Answer from the drawing. Dimensions are ordinates in mm from the lowest x, y and z of the part. Coordinates: 2 decimals unless noted, no trailing zeros. Order: outer loops, then holes, each group sorted by start corner. A loop starts at its lowest first (then second) coordinate and runs counter-clockwise, first axis right, second up. Notation, with made-up numbers: (71.5, 78) - (95.5, 78) arc R17 ccw to (95.5, 84) - close; hole circle Ø10 at (58.5, 27.25). An arc over 180 degrees is marked (long way). Answer as a JSON object with one key per item and string values. Group by question number.
1) Each of these flat-tipped pins is pushed along its axis until it touches: P1, Ø1, axis at y = 164.5, z = 21.5, coming from the -X side; P2, Ø3, axis at x = 309, z = 97, coming from the +Y side. Where does it stop, or does it pass through?
2) Find the intervals of material crossed by line 1 along X through (y, z) = (95.5, 60); line 2 along Z through (x, y) = (65.5, 40.5), in increasing order.
3) Section A-A (x = 300) is taken. Give the vertices of the cut face in (y, z), plus the area to 3 significant figures.
4) Section D-D (x = 158) is taken. Give the vertices of the cut face in (y, z), plus the area to 3 significant figures.
5) Section C-C (y = 100) is taken. Give the vertices of the cut face in (x, z).
6) Section B-B (z = 117) is taken. Give the vertices of the cut face in (x, y).
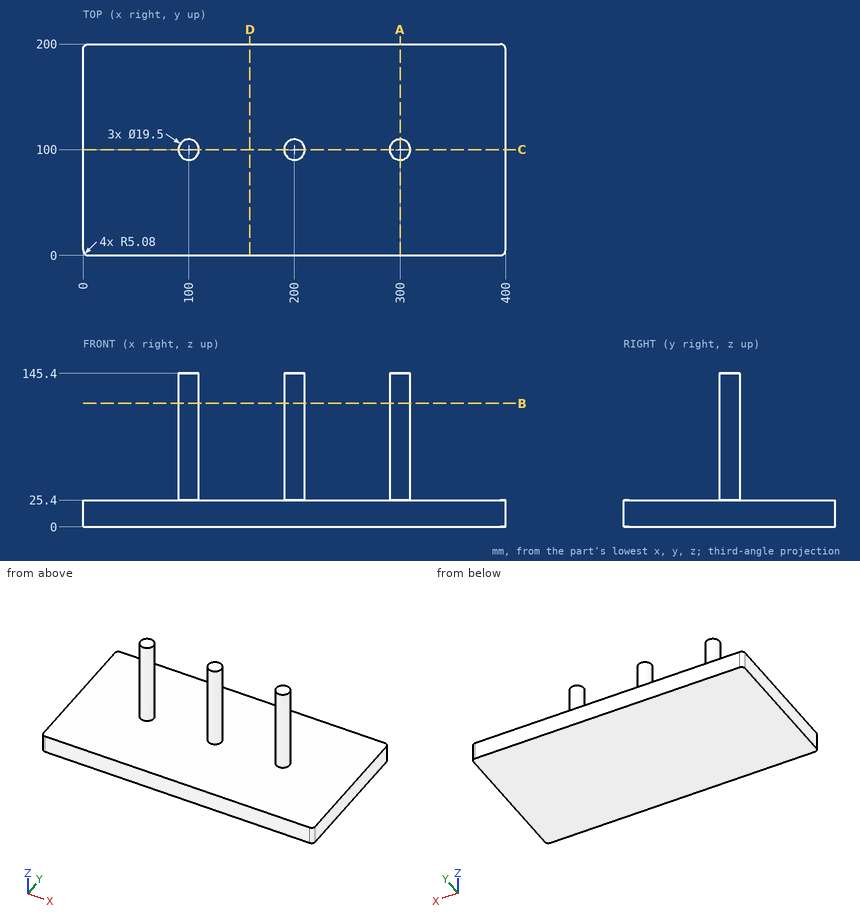
Report:
{
 "1": {"P1": "stops at x = 0", "P2": "stops at y = 106.23"},
 "2": {"line 1": "x = 91.35 to 108.65, 191.35 to 208.65, 291.35 to 308.65", "line 2": "z = 0 to 25.4"},
 "3": {"outline": "(0, 0) - (200, 0) - (200, 25.4) - (109.75, 25.4) - (109.75, 145.4) - (90.25, 145.4) - (90.25, 25.4) - (0, 25.4) - close", "area": "7,420 mm²"},
 "4": {"outline": "(0, 0) - (200, 0) - (200, 25.4) - (0, 25.4) - close", "area": "5,080 mm²"},
 "5": {"outline": "(0, 0) - (400, 0) - (400, 25.4) - (309.75, 25.4) - (309.75, 145.4) - (290.25, 145.4) - (290.25, 25.4) - (209.75, 25.4) - (209.75, 145.4) - (190.25, 145.4) - (190.25, 25.4) - (109.75, 25.4) - (109.75, 145.4) - (90.25, 145.4) - (90.25, 25.4) - (0, 25.4) - close"},
 "6": {"outline": "circle Ø19.5 at (100, 100); circle Ø19.5 at (200, 100); circle Ø19.5 at (300, 100)"}
}
